Geometry: final body of the model. Coordinates: model frame, mm. A direction names the side the tool comes from. Round coordinates to 2 decimals unless told otherwise and drop trailing zeros. Loops run counter-clockwise (first coordinate to the right, second up) from the corner with the lowest first, then second, coordinate; pieces in that order, holes last. Notation, with made-up numbers: (58, 41) - (90, 41) arc R36 cw to (90, 76) - close; hole circle Ø3 at (25, -17). An arc over 180 degrees is marked (long way). Answer as CSV lines item,"result".
from build123d import *

# Parameters (mm, degrees)
F0_W     = 20
F0_H     = 20
F0_R     = 5
F1_DEPTH = 2
F2_W     = 5
F2_H     = 5
F3_DEPTH = 2.001


with BuildPart() as f1:
    # F0 (on Top) → F1 (new body)
    with BuildSketch(Plane.XY):
        Rectangle(F0_W, F0_H)
        Circle(F0_R, mode=Mode.SUBTRACT)
    extrude(amount=F1_DEPTH)

    # F2 (on face) → F3 (cut, through all)
    with BuildSketch(Plane.XY.offset(2)):
        with Locations((-12.5, -5)):
            Rectangle(F2_W, F2_H)
        with Locations((-7.5, -5)):
            Rectangle(F2_W, F2_H)
        with Locations((-12.5, 5)):
            Rectangle(F2_W, F2_H)
        with Locations((-7.5, 5)):
            Rectangle(F2_W, F2_H)
    extrude(amount=-F3_DEPTH, mode=Mode.SUBTRACT)


solid = f1.part
(1) Section D-D (y = -7.25). Output: boundary loops of the cut face in (x, z), and give its area (3 significant figures).
Findings below:
outline,"(-5, 0) - (10, 0) - (10, 2) - (-5, 2) - close"
area,"30.0 mm2"
(2) Draft query along Y for faces 1 (the face through (0, -10, 1)), 2 (the face through (-1.08, -4.88, 0.99)), 3 (the face through (-5, -5, 1)), 4 (the face through (-10, -9, 1)). Return one class per face: pulls with the +Y half, pulls with the -Y half, needs draft (parallel to the pull), parting line crosses it, or undercut.
Findings below:
face 1,"pulls with the -Y half"
face 2,"undercut"
face 3,"undercut"
face 4,"needs draft"
(3) Section A-A (y = 0). Output: boundary loops of the cut face in (x, z).
Findings below:
outline,"(-10, 0) - (-5, 0) - (-5, 2) - (-10, 2) - close; (5, 0) - (10, 0) - (10, 2) - (5, 2) - close"
(4) Section C-C (z = 1.7). Output: boundary loops of the cut face in (x, y), and give its area (3 significant figures).
Findings below:
outline,"(-10, -10) - (10, -10) - (10, 10) - (-10, 10) - (-10, 7.5) - (-5, 7.5) - (-5, 2.5) - (-10, 2.5) - (-10, -2.5) - (-5, -2.5) - (-5, -7.5) - (-10, -7.5) - close; hole circle Ø10 at (0, 0)"
area,"271 mm2"
(5) Access query for faces 5 (the face through (-5, 5, 1)), 6 (the face through (2, 5, 0)). Directions: +Z, -Z, +X, -X, +Y, -Y. A direction counts if a zero-diameter tool reaches every point of the face in a straight line with its end or side. Return the directions, or none.
Findings below:
face 5,"+Z, -Z, -X"
face 6,"-Z, +X, -X, +Y, -Y"
(6) Pin query (flat end, axial travel): P1, Ø1, axis at x = 3, y = 1.5, coming from the +Z side. Return the tip coordinate at first contact, or that it passes through.
Findings below:
P1,"through"
(7) Material intervals for line 1 along Y through (x, z) = (-6, 1.25); line 2 along Y through (x, z) = (0, 0.75); line 3 along Y through (x, z) = (1.75, 1.4), sorted ascending.
Findings below:
line 1,"-10 to -7.5, -2.5 to 2.5, 7.5 to 10"
line 2,"-10 to -5, 5 to 10"
line 3,"-10 to -4.68, 4.68 to 10"
